Check sheet for the modelled part. Datum: model origin and axes. Units: mm. A direction names the side the tool comes from. Give positions to 0.01 mm unless a question says otherwise; leave off trailing zeros. Write each loop counter-clockwise with the first axis right and the second up, starting at its lowest first coordinate (ties: lowest second). Pieces come first, ordered by that corner, then holes. Notation, with made-up numbers: (82, 75.25) -> (113, 75.25) arc R25 cw to (113, 101.25) -> close; hole circle Ø8 at (38, 83.25). An arc over 180 degrees is marked (long way). Answer as a JSON object with one key per item and string values.
from build123d import *

# Parameters (mm, degrees)
BOSS_EXTRUDE1_DEPTH        = 25
F_10_0MM_DOWEL_HOLE1_D     = 10
F_10_0MM_DOWEL_HOLE1_DEPTH = 25
M8_TAPPED_HOLE1_D          = 6.8
M8_TAPPED_HOLE1_DEPTH      = 15


# Read off the part's stored shape, not the designer's step: CSK for M6 Countersunk Flat Head Screw1
with BuildPart() as part:
    # Sketch1 → Boss-Extrude1 (new, symmetric)
    with BuildSketch(Plane.XY):
        Polygon((0, 0), (0, 97), (-44, 97), (-44, 84), (-38, 84), (-38, 90), (-32, 90), (-32, 0), align=None)
    extrude(amount=BOSS_EXTRUDE1_DEPTH, both=True)

    # Ø10.0mm Dowel Hole1
    with Locations(Plane.XY.offset(25)):
        with Locations((-16, 45)):
            Hole(F_10_0MM_DOWEL_HOLE1_D / 2, depth=F_10_0MM_DOWEL_HOLE1_DEPTH)

    # M8 Tapped Hole1
    with Locations(Plane(origin=(0, 0, 0), x_dir=(-1, 0, 0), z_dir=(0, -1, 0))):
        with Locations((7, 0), (25, 0)):
            Hole(M8_TAPPED_HOLE1_D / 2, depth=M8_TAPPED_HOLE1_DEPTH)

    # CSK for M6 Countersunk Flat Head Scr 2 → CSK for M6 Countersunk Flat Head Screw1 (revolve, cut)
    with BuildSketch(Plane(origin=(0, 45, 9), x_dir=(0, 1, 0), z_dir=(0, 0, -1))):
        Polygon((0, -12.244302381), (3.3, -12.244302381), (3.3, -3), (6.3, 0), (0, 0), align=None)
    revolve(axis=Axis((0, 45, 9), (1, 0, 0)), mode=Mode.SUBTRACT)


solid = part.part
1. Sectioned sample at B-B, the plane x = -7. Enter the section's corners in (y, z), plus the area to 3 significant figures.
Determined:
{"outline": "(0, -25) -> (97, -25) -> (97, 25) -> (0, 25) -> (0, 3.4) -> (15, 3.4) -> (15, -3.4) -> (0, -3.4) -> close; hole circle Ø6.6 at (45, 9)", "area": "4,710 mm^2"}
2. Sectioned sample at C-C, the plane y = 45. Enter the section's corners in (x, z).
Determined:
{"outline": "(-32, -25) -> (0, -25) -> (0, 2.7) -> (-3, 5.7) -> (-11, 5.7) -> (-11, 0) -> (-21, 0) -> (-21, 25) -> (-32, 25) -> close; (-11, 12.3) -> (-3, 12.3) -> (0, 15.3) -> (0, 25) -> (-11, 25) -> close"}
3. Sectioned sample at D-D, the plane z = 9. Enter the section's corners in (x, y).
Determined:
{"outline": "(-44, 84) -> (-38, 84) -> (-38, 90) -> (-32, 90) -> (-32, 0) -> (0, 0) -> (0, 38.7) -> (-3, 41.7) -> (-12.24, 41.7) arc R5 cw (long way) to (-12.24, 48.3) -> (-3, 48.3) -> (0, 51.3) -> (0, 97) -> (-44, 97) -> close"}
4. Mould release check, pull along Y, two halves, no side actions. Record for faces 1 (the face through (-7.56, 44.28, 5.78)), 2 (the face through (-25, 15, 0)), 3 (the face through (-2.812, 41.516, 9.153)), 4 (the face through (-12.5, 49.2, 25)): released by +Y, released by -Y, zero draft, split by the parting line, or undercut.
Determined:
{"face 1": "undercut", "face 2": "released by -Y", "face 3": "undercut", "face 4": "zero draft"}
5. Go/stop test with flat-tipped pins: P1, Ø1, axis at x = -39.5, z = 13.5, coming from the -Y side; P2, Ø8.5, axis at y = 45, z = 9, coming from the -X side; P3, Ø3.5, axis at x = -7.5, z = -0.5, coming from the -Y side. Record where each tip stops, or that it passes through.
Determined:
{"P1": "y = 84", "P2": "x = -32", "P3": "y = 15"}
6. Sectioned sample at A-A, the plane z = 16.5. Enter the section's corners in (x, y).
Determined:
{"outline": "(-44, 84) -> (-38, 84) -> (-38, 90) -> (-32, 90) -> (-32, 0) -> (0, 0) -> (0, 97) -> (-44, 97) -> close; hole circle Ø10 at (-16, 45)"}
7. Access from +Z, -Z, +X, -X, +Y, -Y to the whole of each face (thin tool, end or side, straight path). Record for faces 5 (the face through (-35, 90, 0)), 6 (the face through (-3.86, 7.6, 1.3)), 7 (the face through (-20.77, 46.5, 12.33)).
Determined:
{"face 5": "+Z, -Z, -Y", "face 6": "-Y", "face 7": "+Z"}
8. Scan lines: L1, parallel to Y at x = -16, z = 17; L2, parallel to Z at x = -9, y = 45; L3, parallel to X at y = 8.5, z = -18.5. Record each from-to range of solid material in increasing order. Write a range as [from, to].
Determined:
{"L1": "[0, 40], [50, 97]", "L2": "[-25, 5.7], [12.3, 25]", "L3": "[-32, 0]"}
